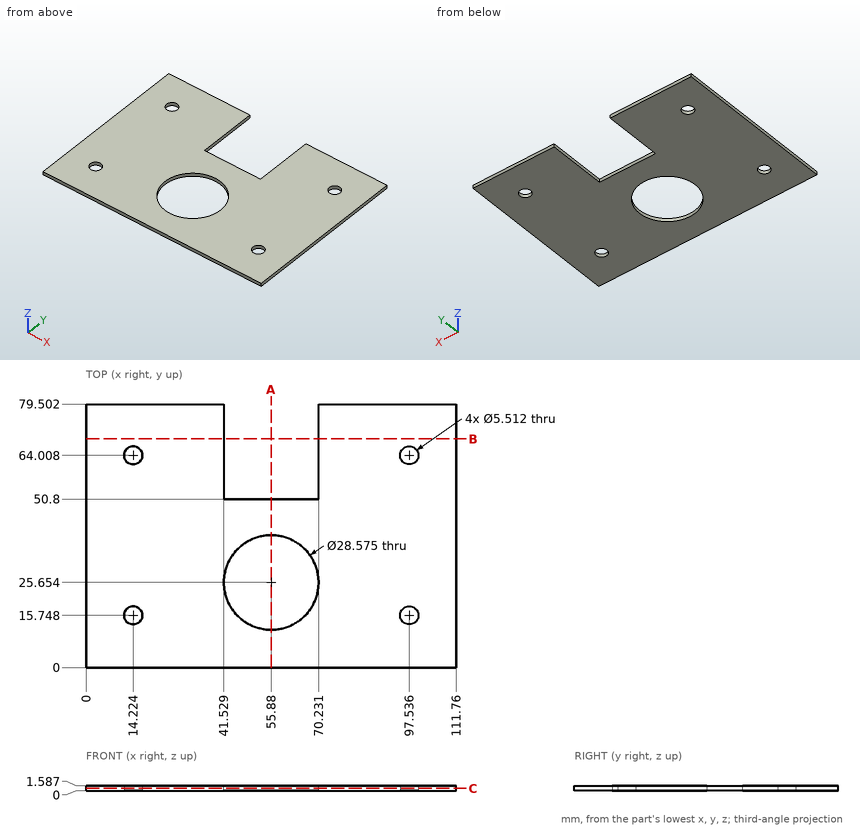
Input: dimensioned drawing with shaded views. Units: mm. Origin: part minimum x, y, z. Coordinates: 2 decimals unless noted, no trailing zeros. Write each loop counter-clockwise with the first axis right and the second up, starting at its lowest first coordinate (ties: lowest second). Pieces come first, ordered by that corner, then holes. Notation, with made-up numbers: M 39,0.25 L 96,0.25 A7 cw 96,11.25 Z; hole C -24.5,-24 d6. An arc over 180 degrees is marked long. Use one line per item in the form item = value.
Q1. Section B-B (y = 69). Return loops of the section in (x, z).
Answer below:
outline = M 0,0 L 41.53,0 L 41.53,1.59 L 0,1.59 Z; M 70.23,0 L 111.76,0 L 111.76,1.59 L 70.23,1.59 Z
Q2. Section A-A (x = 55.88). Return loops of the section in (y, z).
Answer below:
outline = M 0,0 L 11.37,0 L 11.37,1.59 L 0,1.59 Z; M 39.94,0 L 50.8,0 L 50.8,1.59 L 39.94,1.59 Z
Q3. First-contact query: pin 1 (5 mm diameter, centred on x = 14.224, y = 64.008, fed in from +Z). Flat tip, straight axial feed; report the tip coordinate or a pass-through.
Answer below:
pin_1 = through
Q4. Material intervals for probe 1 along Y at (x, z) = (55.88, 0.4); probe 2 along X at (y, z) = (72, 0.3); probe 3 along Y at (x, z) = (59, 0.4), sorted ascending. Write a range as from..to.
Answer below:
probe_1 = 0..11.37, 39.94..50.8
probe_2 = 0..41.53, 70.23..111.76
probe_3 = 0..11.71, 39.6..50.8
Q5. Section C-C (z = 0.75). Return loops of the section in (x, y) (1 decimal).
Answer below:
outline = M 0,0 L 111.8,0 L 111.8,79.5 L 70.2,79.5 L 70.2,50.8 L 41.5,50.8 L 41.5,79.5 L 0,79.5 Z; hole C 14.2,15.7 d5.5; hole C 14.2,64 d5.5; hole C 55.9,25.7 d28.6; hole C 97.5,15.7 d5.5; hole C 97.5,64 d5.5
